from build123d import *

# Parameters (mm, degrees)
CROQUIS1_W              = 72
CROQUIS1_H              = 47
SALIENTE_EXTRUIR1_DEPTH = 1.5
CROQUIS2_R              = 1.6
CORTAR_EXTRUIR1_DEPTH   = 2.5
REDONDEO1_R             = 4
CROQUIS3_W              = 5.75
CROQUIS3_H              = 3.25
CROQUIS3_W_2            = 3.25
CROQUIS3_H_2            = 5.75
CROQUIS3_W_3            = 8
CROQUIS3_H_3            = 8
SALIENTE_EXTRUIR2_DEPTH = 8
CROQUIS6_R              = 2
CROQUIS6_W              = 7.5
CROQUIS6_H              = 8.749690514
CROQUIS6_W_2            = 5
CROQUIS6_H_2            = 3
CROQUIS6_W_3            = 6.25
CROQUIS6_H_3            = 4.5
CROQUIS6_W_4            = 24.5
CROQUIS6_H_4            = 16
SALIENTE_EXTRUIR3_DEPTH = 3


with BuildPart() as part:
    # Croquis1 → Saliente-Extruir1 (new body)
    with BuildSketch(Plane(origin=(0, 0, 0), x_dir=(1, 0, 0), z_dir=(0, 1, 0))):
        Rectangle(CROQUIS1_W, CROQUIS1_H)
    extrude(amount=SALIENTE_EXTRUIR1_DEPTH)

    # Croquis2 → Cortar-Extruir1 (cut, through all)
    with BuildSketch(Plane(origin=(0, 1.5, 0), x_dir=(1, 0, 0), z_dir=(0, 1, 0))):
        with Locations((-32, 19.5)):
            Circle(CROQUIS2_R)
        with Locations((32, 19.5)):
            Circle(CROQUIS2_R)
        with Locations((32, -19.5)):
            Circle(CROQUIS2_R)
        with Locations((-32, -19.5)):
            Circle(CROQUIS2_R)
    extrude(amount=-CORTAR_EXTRUIR1_DEPTH, mode=Mode.SUBTRACT)

    # Redondeo1
    redondeo1_edges = [part.edges().sort_by_distance(p)[0] for p in [
        (36, 0.75, 23.5),
        (-36, 0.75, 23.5),
        (-36, 0.75, -23.5),
        (36, 0.75, -23.5),
    ]]
    fillet(redondeo1_edges, radius=REDONDEO1_R)

    # Croquis3 → Saliente-Extruir2 (add)
    with BuildSketch(Plane(origin=(0, 1.5, 0), x_dir=(1, 0, 0), z_dir=(0, 1, 0))):
        Polygon((-4.1, 11.25), (-7.2, 11.25), (-7.2, 13.75), (-26.1, 13.75), (-26.1, 22.25), (-4.1, 22.25), align=None)
        with Locations((9.025, -18.875)):
            Rectangle(CROQUIS3_W, CROQUIS3_H)
        with Locations((9.025, 18.875)):
            Rectangle(CROQUIS3_W, CROQUIS3_H)
        Polygon((-7.2, -13.75), (-26.1, -13.75), (-26.1, -22.25), (-4.1, -22.25), (-4.1, -11.25), (-7.2, -11.25), align=None)
        with Locations((25.375, 10.625)):
            Rectangle(CROQUIS3_W_2, CROQUIS3_H_2)
        with Locations((31.5, 10.625)):
            Rectangle(CROQUIS3_W_3, CROQUIS3_H_3)
        with Locations((6.5, 0)):
            Rectangle(CROQUIS3_W_3, CROQUIS3_H)
    extrude(amount=SALIENTE_EXTRUIR2_DEPTH)

    # Croquis6 → Saliente-Extruir3 (add)
    with BuildSketch(Plane(origin=(0, 1.5, 0), x_dir=(1, 0, 0), z_dir=(0, 1, 0))):
        with Locations((-1.3, 0)):
            Circle(CROQUIS6_R)
        with Locations((32.25, -4.749845257)):
            Rectangle(CROQUIS6_W, CROQUIS6_H)
        with Locations((17.248785916, -20.25)):
            Rectangle(CROQUIS6_W_2, CROQUIS6_H_2)
        with Locations((24.5, -20.25)):
            Rectangle(CROQUIS6_W_2, CROQUIS6_H_2)
        with Locations((1.875, 20.5)):
            Rectangle(CROQUIS6_W_3, CROQUIS6_H_3)
        with Locations((-21.75, 0)):
            Rectangle(CROQUIS6_W_4, CROQUIS6_H_4)
    extrude(amount=SALIENTE_EXTRUIR3_DEPTH)


solid = part.part
Here's how the part is built. I have some questions about the finished solid (model axes, mm). A direction names the side the tool comes from. Coordinates: 2 decimals unless noted, no trailing zeros. Order: outer loops, then holes, each group sorted by start corner. A loop starts at its lowest first (then second) coordinate and runs counter-clockwise, first axis right, second up.
Item 1: If we section it at A-A on z = -12: List the corners of the cut face in (x, y) for me.
Result sheet:
outline: (-36, 0) - (36, 0) - (36, 1.5) - (35.5, 1.5) - (35.5, 9.5) - (27.5, 9.5) - (27.5, 1.5) - (27, 1.5) - (27, 9.5) - (23.75, 9.5) - (23.75, 1.5) - (-4.1, 1.5) - (-4.1, 9.5) - (-7.2, 9.5) - (-7.2, 1.5) - (-36, 1.5) - close
Item 2: If we mould it in two halves opening along X, with no side actions, what happens to faces 1 (the face through (22, 3, 20)), 2 (the face through (-33.18, 0.76, 18.42)), 3 (the face through (-15, 9.5, -18)), 4 (the face through (-7.2, 5, -12))? For each: +X half, -X half, draft (parallel to the pull), parting line (faces both ways), or undercut.
Result sheet:
face 1: undercut
face 2: undercut
face 3: draft
face 4: -X half
Item 3: For faces 5 (the face through (17, 4.5, 20)), 6 (the face through (24, 3, 21.75)), 7 (the face through (6.15, 5, -19)), 8 (the face through (9, 5, 17.25)), 9 (the face through (31, 5, -14.625)), which set-ups out of +Z, -Z, +X, -X, +Y, -Y let a thin tool reach every point of the face, with its end or its side?
Result sheet:
face 5: +Z, -Z, +X, +Y
face 6: +Z, +X, +Y
face 7: -Z, +Y
face 8: +X, +Y
face 9: -Z, +X, +Y
Item 4: I need wall thicknesses on line 1 (X direction, y = 0.9, z = -19.5); line 2 (Z direction, x = 32, y = 1); line 3 (X direction, y = 9, z = -12). Which ranges of each line are inside material? Lowest first, please.
Result sheet:
line 1: x = -36 to -33.6, -30.4 to 30.4, 33.6 to 36
line 2: z = -23.5 to -21.1, -17.9 to 17.9, 21.1 to 23.5
line 3: x = -7.2 to -4.1, 23.75 to 27, 27.5 to 35.5
Item 5: For P1, Ø8, axis at x = 19, z = 3.5, coming from the -Y side; P2, Ø5, axis at x = 32, z = 19.5, coming from the +Y side; P3, Ø8, axis at x = -18, z = -0.5, coming from the +Y side; P4, Ø4, axis at x = 31, y = 5, coming from the -Z side (3 decimals), each with a flat end and sliding along its axis, tell me the tip position at first contact or that it passes through.
Result sheet:
P1: stops at y = 0
P2: stops at y = 1.5
P3: stops at y = 4.5
P4: stops at z = -14.625
Item 6: If we section it at B-B on x = -15: List the corners of the cut face in (y, z) for me, plus the area to 4 significant figures.
Result sheet:
outline: (0, -23.5) - (1.5, -23.5) - (1.5, -22.25) - (9.5, -22.25) - (9.5, -13.75) - (1.5, -13.75) - (1.5, -8) - (4.5, -8) - (4.5, 8) - (1.5, 8) - (1.5, 13.75) - (9.5, 13.75) - (9.5, 22.25) - (1.5, 22.25) - (1.5, 23.5) - (0, 23.5) - close
area: 254.5 mm2
